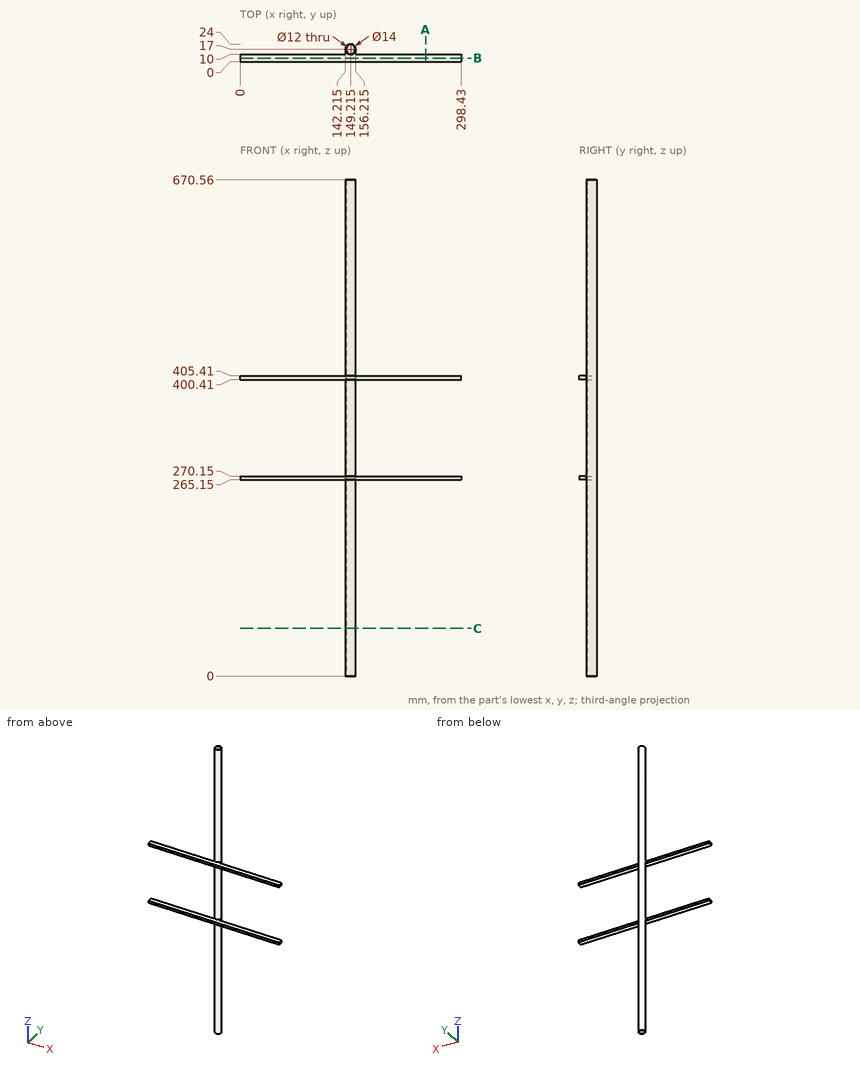
Job drawing, mm, ordinate dimensions from the low corner. One solid piece. Coordinates: 2 decimals unless noted, no trailing zeros. Loops run counter-clockwise (first coordinate to the right, second up) from the corner with the lowest first, then second, coordinate; pieces in that order, holes last. Notation, with made-up numbers: (-8, 87.25) - (18, 87.25) arc R16 cw to (18, 106.25) - close; hole circle Ø11 at (67.25, -28.75). An arc over 180 degrees is marked (long way). Write item = value, one per line. Start each with the question number.
Q1. Flat gauge pins, fed straight in: pin 1 Ø1.5 at (y, z) = (12.5, 403) entering from -X (3 decimals); pin 2 Ø1.5 at (x, z) = (235, 403) entering from +Y; pin 3 Ø10 at (x, y) = (140, 5) entering from -Z. Where does each tip first touch, or does it go through?
Q2. Cut at A-A, the plane x = 250.5. List the corners of the cut face in (y, z), then the cut area to 3 significant figures.
Q3. Drill centre lines: L1, parallel to X at y = 18.25, z = 630.5; L2, parallel to Z at x = 18.5, y = 9.75; L3, parallel to X at y = 16.25, z = 332.5. Where is each one in solid material? Low to high.
Q4. Cut at C-C, the plane z = 64.5. List the corners of the cut face in (x, y) (3 decimals), then the cut area to 3 significant figures.
Q5. Cut at B-B, the plane y = 5. List the corners of the cut face in (x, z).
Computed:
q1.pin_1 = 142.215
q1.pin_2 = 10
q1.pin_3 = 265.15
q2.outline = (0, 265.15) - (10, 265.15) - (10, 270.15) - (0, 270.15) - close; (0, 400.41) - (10, 400.41) - (10, 405.41) - (0, 405.41) - close
q2.area = 100 mm²
q3.L1 = 142.33 to 143.35, 155.08 to 156.1
q3.L2 = 265.15 to 270.15, 400.41 to 405.41
q3.L3 = 142.26 to 143.26, 155.17 to 156.17
q4.outline = circle Ø14 at (149.215, 17); hole circle Ø12 at (149.215, 17)
q4.area = 40.8 mm²
q5.outline = (0, 265.15) - (298.43, 265.15) - (298.43, 270.15) - (0, 270.15) - close; (0, 400.41) - (298.43, 400.41) - (298.43, 405.41) - (0, 405.41) - close
